from build123d import *

# Parameters (mm, degrees)
F1_DEPTH = 50.8
F2_DEPTH = 50.8
F5_T     = -6.35
F4_W     = 38.1
F4_H     = 88.9
F6_DEPTH = 31.75


with BuildPart() as f1:
    # F0 (on Front) → F1 (new body)
    with BuildSketch(Plane.XZ):
        Polygon((24.13, -15.24), (24.13, 15.24), (19.05, 15.24), (19.05, -10.16), (-19.05, -10.16), (-19.05, 15.24), (-24.13, 15.24), (-24.13, -15.24), align=None)
    extrude(amount=F1_DEPTH)

    # F0 (on Front) → F2 (join)
    with BuildSketch(Plane.XZ):
        Polygon((19.05, -10.16), (19.05, 15.24), (3.175, 15.24), (3.175, 8.8727482983), (-3.175, 8.8727482983), (-3.175, 15.24), (-19.05, 15.24), (-19.05, -10.16), align=None)
    extrude(amount=F2_DEPTH)

    # F3: F1 across plane


with BuildPart() as f1_1:
    add(f1.part)
    add(f1.part.mirror(Plane.XZ))

    # F5
    f5_openings = [f1_1.faces().sort_by_distance(p)[0] for p in [
        (13.6525, 0, 15.24),
        (-13.6525, 0, 15.24),
    ]]
    offset(amount=F5_T, openings=f5_openings, kind=Kind.INTERSECTION)

    # F4 (on Top) → F6 (cut)
    with BuildSketch(Plane.XY):
        Rectangle(F4_W, F4_H)
    extrude(amount=F6_DEPTH, mode=Mode.SUBTRACT)


solid = f1_1.part
Work out the finished part from the listing and answer in its coordinate system (mm). A direction names the side the tool comes from. Round coordinates to 2 decimals unless told otherwise and drop trailing zeros. Order: outer loops, then holes, each group sorted by start corner. A loop starts at its lowest first (then second) coordinate and runs counter-clockwise, first axis right, second up. Notation, with made-up numbers: M 69.5,9 L 112.5,9 A23 ccw 112.5,44 Z; hole C -30.75,27 d9. An arc over 180 degrees is marked long. Put each result on its own line as item: value. Start each with the question number.
Q1. Section C-C, the plane x = -9 is taken. Write down the section's boundary in (y, z), and give its area (3 significant figures).
Q2. Section A-A, the plane z = 11 is taken. Write down the section's boundary in (x, y) (3 decimals).
Q3. Section D-D, the plane y = 13.5 is taken. Write down the section's boundary in (x, z), and give its area (3 significant figures).
Q4. A tool of negligible diameter and unlimited length cuts with its end or side. For faces 1 (the flat face through (-3.175, -48, 12)), 2 (the flat face through (-24.13, -1, 0)), 3 (the flat face through (17.78, -1, -5)), from which of +Z, -Z, +X, -X, +Y, -Y can it reach the whole face along a straight path? Write none if from no direction.
Q5. For a pull along Y with two mould halves and no side action, classify faces 4 (the flat face through (-3.175, 48, 12)), 5 (the flat face through (0, -44.45, 3)), 6 (the flat face through (0, 50.8, 0)) as pulls with the +Y half, pulls with the -Y half, needs draft (parallel to the pull), parting line crosses it, or undercut.
Q6. Flat-ended cylindrical pins translate along their axes: pin 1 (3 mm diameter, centred on x = 14, y = 21.5, fed in from +Z); pin 2 (5 mm diameter, centred on x = 1, y = 47.5, fed in from +Z); pin 3 (3 mm diameter, centred on x = 1.5, y = -47.5, fed in from +Z). Find the tip coordinate at first contact, or state that the pin passes through.
Q7. Section B-B, the plane z = -5.5 is taken. Write down the section's boundary in (x, y), and give its area (3 significant figures).
Q8. Straight lines are drawn through the part: L1, parallel to X at y = -27, z = 13; L2, parallel to X at y = -25, z = -3.5; L3, parallel to Y at x = -17.5, z = 4. For each, find the intervals that lie inside material, in ascending order. Write a range as [from, to].
Findings below:
1. outline: M -50.8,-15.24 L 50.8,-15.24 L 50.8,15.24 L 44.45,15.24 L 44.45,-8.89 L -44.45,-8.89 L -44.45,15.24 L -50.8,15.24 Z
1. area: 952 mm^2
2. outline: M -24.13,-50.8 L -3.175,-50.8 L -3.175,-44.45 L -19.05,-44.45 L -19.05,44.45 L -3.175,44.45 L -3.175,50.8 L -24.13,50.8 Z; M 3.175,-50.8 L 24.13,-50.8 L 24.13,50.8 L 3.175,50.8 L 3.175,44.45 L 19.05,44.45 L 19.05,-44.45 L 3.175,-44.45 Z
3. outline: M -24.13,-15.24 L 24.13,-15.24 L 24.13,15.24 L 19.05,15.24 L 19.05,0 L 17.78,0 L 17.78,-8.89 L -17.78,-8.89 L -17.78,0 L -19.05,0 L -19.05,15.24 L -24.13,15.24 Z
3. area: 574 mm^2
4. face 1: +Z, +Y, -Y
4. face 2: +Z, -Z, -X, +Y, -Y
4. face 3: +Z
5. face 4: needs draft
5. face 5: undercut
5. face 6: pulls with the +Y half
6. pin 1: stops at z = -8.89
6. pin 2: stops at z = 15.24
6. pin 3: stops at z = 8.87
7. outline: M -24.13,-50.8 L 24.13,-50.8 L 24.13,50.8 L -24.13,50.8 Z; hole M -17.78,-44.45 L 17.78,-44.45 L 17.78,44.45 L -17.78,44.45 Z
7. area: 1,740 mm^2
8. L1: x = [-24.13, -19.05], [19.05, 24.13]
8. L2: x = [-24.13, -17.78], [17.78, 24.13]
8. L3: y = [-50.8, -44.45], [44.45, 50.8]
